Source: CAD feature listing. Evaluate the final solid. Frame: model axes, mm. Face numbers are marked on the shaded views. A direction names the side the tool comes from. Give positions to 0.01 mm unless a question says otherwise; leave off trailing zeros.
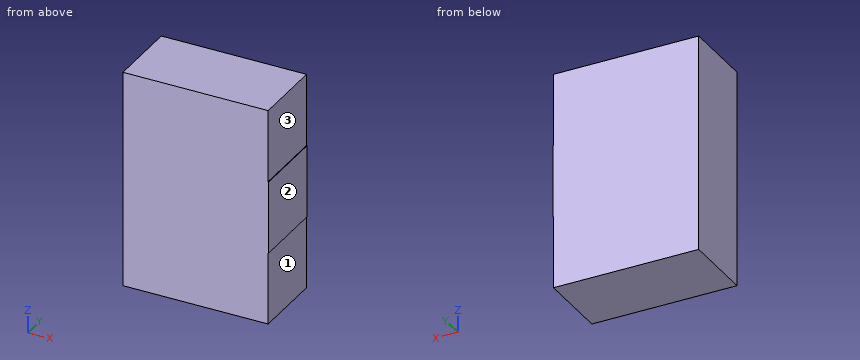
from build123d import *

# Parameters (mm, degrees)
F0_W     = 25.4
F0_H     = 25.4
F1_DEPTH = 25.4


with BuildPart() as f1:
    # F0 (on Front) → F1 (new body)
    with BuildSketch(Plane.XZ):
        with Locations((12.7, 12.7)):
            Rectangle(F0_W, F0_H)
        with Locations((-12.7, 12.7)):
            Rectangle(F0_W, F0_H)
        with Locations((-12.7, -12.7)):
            Rectangle(F0_W, F0_H)
        Polygon((25.4, 0), (0, 0), (0, -25.4), (25.4, -25.4), (25.591951, -25.4), (25.591951, 0), align=None)
        with Locations((-12.7, -38.1)):
            Rectangle(F0_W, F0_H)
        with Locations((12.7, -38.1)):
            Rectangle(F0_W, F0_H)
    extrude(amount=F1_DEPTH)


solid = f1.part
1) Reachability of the marked faces 1, 2 and 3 from +Z, -Z, +X, -X, +Y, -Y: full face, straight path, thin tool, end or side. Return the list, or none.
Checks:
face 1: -Z, +X, +Y, -Y
face 2: +Z, -Z, +X, +Y, -Y
face 3: +Z, +X, +Y, -Y
2) Ray query, probe 1 along X at (y, z) = (-10.25, -45). Return the intervals inside material, ascending.
Checks:
probe 1: x = -25.4 to 25.4
3) Contact query for a flat-ended pin moving along its axis: P1, Ø12.5, axis at y = -16, z = 9, coming from the +X side. Output: stop coordinate, or through.
Checks:
P1: stops at x = 25.4
